from build123d import *

# Parameters (mm, degrees)
SALIENTE_EXTRUIR1_DEPTH = 10
VACIADO2_START          = -40.8
VACIADO2_OUTLINE_W      = 121.6
VACIADO2_OUTLINE_H      = 9.4
VACIADO2_DEPTH          = 81.6
VACIADO2_START_2        = -49.5
VACIADO2_2_OUTLINE_W    = 49.4
VACIADO2_2_OUTLINE_H    = 9.4
VACIADO2_2_DEPTH        = 99
VACIADO2_3_OUTLINE_W    = 8.7
VACIADO2_3_OUTLINE_H    = 9.4
VACIADO2_3_DEPTH        = 38.1
VACIADO2_START_3        = 11.4
VACIADO2_4_OUTLINE_W    = 8.7
VACIADO2_4_OUTLINE_H    = 9.4
VACIADO2_4_DEPTH        = 38.1
SALIENTE_EXTRUIR6_DEPTH = 0.3


# Read off the part's stored shape, not the designer's step: Vaciado2
with BuildPart() as part:
    # Croquis1 → Saliente-Extruir1 (new body)
    with BuildSketch(Plane(origin=(0, 0, 0), x_dir=(1, 0, 0), z_dir=(0, 1, 0))):
        Polygon((-11.3, -50), (-11.3, -58.3), (-16.3, -58.3), (-16.3, -61.7), (-11.3, -61.7), (-11.3, -66.3), (11.3, -66.3), (11.3, -61.7), (16.3, -61.7), (16.3, -58.3), (11.3, -58.3), (11.3, -50), (70, -50), (70, -11.3), (78.3, -11.3), (78.3, -16.3), (81.7, -16.3), (81.7, -11.3), (86.3, -11.3), (86.3, 11.3), (81.7, 11.3), (81.7, 16.3), (78.3, 16.3), (78.3, 11.3), (70, 11.3), (70, 50), (11.3, 50), (11.3, 58.3), (16.3, 58.3), (16.3, 61.7), (11.3, 61.7), (11.3, 66.3), (-11.3, 66.3), (-11.3, 61.7), (-16.3, 61.7), (-16.3, 58.3), (-11.3, 58.3), (-11.3, 50), (-70, 50), (-70, 11.3), (-78.3, 11.3), (-78.3, 16.3), (-81.7, 16.3), (-81.7, 11.3), (-86.3, 11.3), (-86.3, -11.3), (-81.7, -11.3), (-81.7, -16.3), (-78.3, -16.3), (-78.3, -11.3), (-70, -11.3), (-70, -50), align=None)
        Polygon((-10.9, 41.3), (-10.9, 58.7), (-15.9, 58.7), (-15.9, 61.3), (-10.9, 61.3), (-10.9, 65.9), (10.9, 65.9), (10.9, 61.3), (15.9, 61.3), (15.9, 58.7), (10.9, 58.7), (10.9, 41.3), align=None, mode=Mode.SUBTRACT)
        Polygon((-10.9, -41.3), (10.9, -41.3), (10.9, -58.7), (15.9, -58.7), (15.9, -61.3), (10.9, -61.3), (10.9, -65.9), (-10.9, -65.9), (-10.9, -61.3), (-15.9, -61.3), (-15.9, -58.7), (-10.9, -58.7), align=None, mode=Mode.SUBTRACT)
        Polygon((-61.3, -10.9), (-78.7, -10.9), (-78.7, -15.9), (-81.3, -15.9), (-81.3, -10.9), (-85.9, -10.9), (-85.9, 10.9), (-81.3, 10.9), (-81.3, 15.9), (-78.7, 15.9), (-78.7, 10.9), (-61.3, 10.9), align=None, mode=Mode.SUBTRACT)
        Polygon((61.3, -10.9), (61.3, 10.9), (78.7, 10.9), (78.7, 15.9), (81.3, 15.9), (81.3, 10.9), (85.9, 10.9), (85.9, -10.9), (81.3, -10.9), (81.3, -15.9), (78.7, -15.9), (78.7, -10.9), align=None, mode=Mode.SUBTRACT)
    extrude(amount=-SALIENTE_EXTRUIR1_DEPTH)

    # Vaciado2 outline → Vaciado2 (cut)
    with BuildSketch(Plane.XY.offset(VACIADO2_START)):
        with Locations((0, -4.7)):
            Rectangle(VACIADO2_OUTLINE_W, VACIADO2_OUTLINE_H)
    extrude(amount=VACIADO2_DEPTH, mode=Mode.SUBTRACT)

    # Vaciado2 2 outline → Vaciado2 2 (cut)
    with BuildSketch(Plane.XY.offset(VACIADO2_START_2)):
        with Locations((-36.1, -4.7)):
            Rectangle(VACIADO2_2_OUTLINE_W, VACIADO2_2_OUTLINE_H)
        with Locations((36.1, -4.7)):
            Rectangle(VACIADO2_2_OUTLINE_W, VACIADO2_2_OUTLINE_H)
    extrude(amount=VACIADO2_2_DEPTH, mode=Mode.SUBTRACT)

    # Vaciado2 3 outline → Vaciado2 3 (cut)
    with BuildSketch(Plane.XY.offset(VACIADO2_START_2)):
        with Locations((-65.15, -4.7)):
            Rectangle(VACIADO2_3_OUTLINE_W, VACIADO2_3_OUTLINE_H)
        with Locations((65.15, -4.7)):
            Rectangle(VACIADO2_3_OUTLINE_W, VACIADO2_3_OUTLINE_H)
    extrude(amount=VACIADO2_3_DEPTH, mode=Mode.SUBTRACT)

    # Vaciado2 4 outline → Vaciado2 4 (cut)
    with BuildSketch(Plane.XY.offset(VACIADO2_START_3)):
        with Locations((-65.15, -4.7)):
            Rectangle(VACIADO2_4_OUTLINE_W, VACIADO2_4_OUTLINE_H)
        with Locations((65.15, -4.7)):
            Rectangle(VACIADO2_4_OUTLINE_W, VACIADO2_4_OUTLINE_H)
    extrude(amount=VACIADO2_4_DEPTH, mode=Mode.SUBTRACT)

    # Croquis4 → Saliente-Extruir6 (add)
    with BuildSketch(Plane.XZ.offset(10)):
        Polygon((-11.3, 50), (-70, 50), (-70, 11.3), (-78.3, 11.3), (-78.3, 16.3), (-81.7, 16.3), (-81.7, 11.3), (-86.3, 11.3), (-86.3, -11.3), (-81.7, -11.3), (-81.7, -16.3), (-78.3, -16.3), (-78.3, -11.3), (-70, -11.3), (-70, -50), (-11.3, -50), (-11.3, -58.3), (-16.3, -58.3), (-16.3, -61.7), (-11.3, -61.7), (-11.3, -66.3), (11.3, -66.3), (11.3, -61.7), (16.3, -61.7), (16.3, -58.3), (11.3, -58.3), (11.3, -50), (70, -50), (70, -11.3), (78.3, -11.3), (78.3, -16.3), (81.7, -16.3), (81.7, -11.3), (86.3, -11.3), (86.3, 11.3), (81.7, 11.3), (81.7, 16.3), (78.3, 16.3), (78.3, 11.3), (70, 11.3), (70, 50), (11.3, 50), (11.3, 58.3), (16.3, 58.3), (16.3, 61.7), (11.3, 61.7), (11.3, 66.3), (-11.3, 66.3), (-11.3, 61.7), (-16.3, 61.7), (-16.3, 58.3), (-11.3, 58.3), align=None)
    extrude(amount=SALIENTE_EXTRUIR6_DEPTH)


solid = part.part
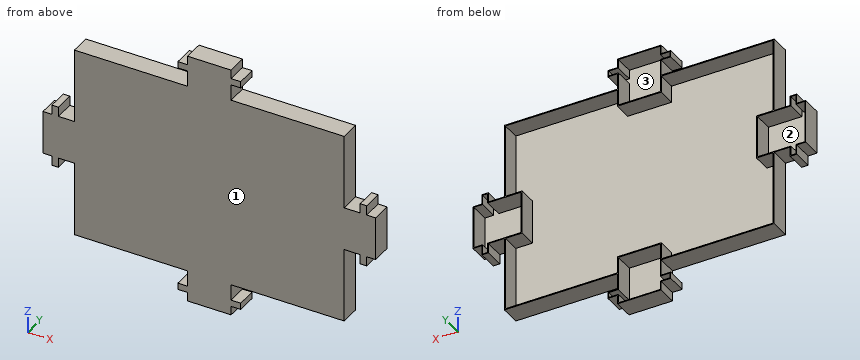
The listing builds one solid part. Answer for the finished solid, in the listing's coordinates (mm). Face numbers are marked on the shaded views. Give positions to 0.01 mm unless a question says otherwise; leave off trailing zeros. Loops run counter-clockwise (first coordinate to the right, second up) from the corner with the lowest first, then second, coordinate; pieces in that order, holes last. Notation, with made-up numbers: (-16.5, 64) - (35.5, 64) arc R23 ccw to (35.5, 76) - close; hole circle Ø5 at (85, 79). An arc over 180 degrees is marked (long way). Use one line per item in the form item = value.
1. Section A-A on z = 29 is taken. Give the vertices of the cut face in (x, y).
Calculated:
outline = (-70, -10.3) - (70, -10.3) - (70, 0) - (69.5, 0) - (69.5, -9.4) - (-69.5, -9.4) - (-69.5, 0) - (-70, 0) - close
2. Section C-C on y = -3.5 is taken. Count the separate pieces of the cut face and the enclosed holes in it, then the cut area to 3 significant figures.
Calculated:
separate_pieces = 1
enclosed_holes = 5
area = 393 mm^2
3. Section D-D on z = -7.5 is taken. Give the vertices of the cut face in (x, y).
Calculated:
outline = (-86.3, -10.3) - (86.3, -10.3) - (86.3, 0) - (85.9, 0) - (85.9, -10) - (61.3, -10) - (61.3, 0) - (60.8, 0) - (60.8, -9.4) - (-60.8, -9.4) - (-60.8, 0) - (-61.3, 0) - (-61.3, -10) - (-85.9, -10) - (-85.9, 0) - (-86.3, 0) - close
4. Find the intervals of material crossed by line 1 along X through (y, z) = (-1.75, 5); line 2 along Z through (x, y) = (-11, -2.5); line 3 along Z through (x, y) = (-67, -7.75), in increasing order. Write a range as [from, to].
Calculated:
line_1 = [-86.3, -85.9], [-61.3, -60.8], [60.8, 61.3], [85.9, 86.3]
line_2 = [-66.3, -61.3], [-58.7, -40.8], [40.8, 58.7], [61.3, 66.3]
line_3 = [-50, -49.5], [-11.4, -10.9], [10.9, 11.4], [49.5, 50]
5. Section B-B on x = -18.5 is taken. Give the vertices of the cut face in (y, z), then the cut area to 3 significant figures.
Calculated:
outline = (-10.3, -50) - (0, -50) - (0, -49.5) - (-9.4, -49.5) - (-9.4, 49.5) - (0, 49.5) - (0, 50) - (-10.3, 50) - close
area = 99.4 mm^2
6. Given pin 1 Ø3.5 at (y, z) = (-5.5, -62.5) entering from -X; pin 2 Ø2.5 at (y, z) = (-3, -13.5) entering from -X; pin 3 Ø5 at (y, z) = (-5.5, 33.5) entering from +X, each flat-ended and moving along its own axis, determine where each tip first touches the part or whether it passes through.
Calculated:
pin_1 = -16.3
pin_2 = -81.7
pin_3 = 70
7. The mould has two halves that part along Z. Classify the marked faces 1, 2 and 3: pulls with the +Z half, pulls with the -Z half, needs draft (parallel to the pull), parting line crosses it, or undercut.
Calculated:
face_1 = needs draft
face_2 = undercut
face_3 = undercut
